Input: part model. Units: mm. Frame: model coordinates. Face numbers are marked on the shaded views. A direction names the side the tool comes from. Round coordinates to 2 decimals unless told otherwise and drop trailing zeros. Loops run counter-clockwise (first coordinate to the right, second up) from the corner with the lowest first, then second, coordinate; pieces in that order, holes last.
(1) Cut plane B-B, the plane x = 26.5. Output: boundary loops of the cut face in (y, z), and give its area (3 significant figures).
(2) Cut plane D-D, the plane x = 8. Output: boundary loops of the cut face in (y, z), and give its area (3 significant figures).
(3) Cut plane A-A, the plane z = -8.5. Output: boundary loops of the cut face in (x, y).
(4) Cut plane C-C, the plane y = 15.5. Output: boundary loops of the cut face in (x, z), and give its area (3 significant figures).
(5) First-contact query: pin 1 Ø3 at (x, y) = (25.5, 24) entering from -Z; pin 2 Ø1.5 at (y, z) = (-6.5, -18.5) entering from -X; pin 3 Ø7 at (y, z) = (22.5, -12) entering from -X. Flat tips, straight axial feed; report the tip coordinate or a pass-through.
(6) Draft query along X for the marked faces 1, 2 and 3. Return one class per face: released by +X, released by -X, zero draft, split by the parting line, or undercut.
(7) Access query for the marked faces 4, 5, 6 and 7. Directions: +Z, -Z, +X, -X, +Y, -Y. A direction counts if a zero-diameter tool reaches every point of the face in a straight line with its end or side. Return the directions, or none.
(8) Line query: line 1 (Y direction, x = 26.5, z = -3.4); line 2 (X direction, y = 7, z = -4); line 3 (X direction, y = 21.5, z = -9.75). Output: solid intervals per line, ascending.
from build123d import *

# Parameters (mm, degrees)
EXTRUDE_1_DEPTH     = 30
FILLET_1_R          = 2
SKETCH_2_W          = 4
SKETCH_2_H          = 30
EXTRUDE_2_DEPTH     = 12
SKETCH_3_W          = 79.384571865
SKETCH_3_H          = 60.739492306
CUT_EXTRUDE_1_DEPTH = 30
SKETCH_4_R          = 1.75
CUT_EXTRUDE_2_DEPTH = 30
SKETCH_5_R          = 3
CUT_EXTRUDE_3_DEPTH = 2
FILLET_2_R          = 2
SKETCH_6_W          = 24
SKETCH_6_H          = 3
EXTRUDE_4_DEPTH     = 12
SKETCH_7_R          = 1.7
CUT_EXTRUDE_4_DEPTH = 12
FILLET_3_R          = 3
FILLET_4_R          = 2


with BuildPart() as part:
    # 草图1 → 凸台-拉伸1 (new body)
    with BuildSketch(Plane(origin=(0, 0, 0), x_dir=(1, 0, 0), z_dir=(0, 1, 0))):
        with BuildLine():
            Line((15.165750888, 20.5), (-15.165750888, 20.5))
            ThreePointArc((-15.165750888, 20.5), (-18.03122292, 18.03122292), (-20.5, 15.165750888))
            Line((-20.5, 15.165750888), (-20.5, -15.165750888))
            ThreePointArc((-20.5, -15.165750888), (-18.03122292, -18.03122292), (-15.165750888, -20.5))
            Line((-15.165750888, -20.5), (15.165750888, -20.5))
            ThreePointArc((15.165750888, -20.5), (18.03122292, -18.03122292), (20.5, -15.165750888))
            Line((20.5, -15.165750888), (20.5, 15.165750888))
            ThreePointArc((20.5, 15.165750888), (18.03122292, 18.03122292), (15.165750888, 20.5))
        make_face()
        with BuildLine():
            Line((-17.5, 14.142135624), (-17.5, -14.142135624))
            ThreePointArc((-17.5, -14.142135624), (-15.909902577, -15.909902577), (-14.142135624, -17.5))
            Line((-14.142135624, -17.5), (14.142135624, -17.5))
            ThreePointArc((14.142135624, -17.5), (15.909902577, -15.909902577), (17.5, -14.142135624))
            Line((17.5, -14.142135624), (17.5, 14.142135624))
            ThreePointArc((17.5, 14.142135624), (15.909902577, 15.909902577), (14.142135624, 17.5))
            Line((14.142135624, 17.5), (-14.142135624, 17.5))
            ThreePointArc((-14.142135624, 17.5), (-15.909902577, 15.909902577), (-17.5, 14.142135624))
        make_face(mode=Mode.SUBTRACT)
    extrude(amount=EXTRUDE_1_DEPTH)

    # 圆角1
    fillet_1_edges = [part.edges().sort_by_distance(p)[0] for p in [
        (-14.142135624, 15, -17.5),
        (-17.5, 15, -14.142135624),
        (-17.5, 15, 14.142135624),
        (-14.142135624, 15, 17.5),
        (14.142135624, 15, 17.5),
        (17.5, 15, 14.142135624),
        (17.5, 15, -14.142135624),
        (14.142135624, 15, -17.5),
    ]]
    fillet(fillet_1_edges, radius=FILLET_1_R)

    # 草图2 → 凸台-拉伸2 (add)
    with BuildSketch(Plane.ZY.offset(20.5)):
        with Locations((-2.25, 15)):
            Rectangle(SKETCH_2_W, SKETCH_2_H)
    extrude_2 = extrude(amount=EXTRUDE_2_DEPTH)

    # 草图3 → 切除-拉伸1 (cut)
    with BuildSketch(Plane.XY.offset(-0.25)):
        with Locations((-5.656839026, 19.40389916)):
            Rectangle(SKETCH_3_W, SKETCH_3_H)
    cut_extrude_1 = extrude(amount=CUT_EXTRUDE_1_DEPTH, mode=Mode.SUBTRACT)

    # 草图4 → 切除-拉伸2 (cut)
    with BuildSketch(Plane(origin=(0, 0, -4.25), x_dir=(-1, 0, 0), z_dir=(0, 0, -1))):
        with Locations(Location((26.5, 23, 0), (0, 0, 90))):
            Circle(SKETCH_4_R)
        with Locations(Location((26.5, 7, 0), (0, 0, 90))):
            Circle(SKETCH_4_R)
    cut_extrude_2 = extrude(amount=-CUT_EXTRUDE_2_DEPTH, mode=Mode.SUBTRACT)

    # 草图5 → 切除-拉伸3 (cut)
    with BuildSketch(Plane(origin=(0, 0, -4.25), x_dir=(-1, 0, 0), z_dir=(0, 0, -1))):
        with Locations(Location((26.5, 23, 0), (0, 0, 90))):
            Circle(SKETCH_5_R)
        with Locations(Location((26.5, 7, 0), (0, 0, 90))):
            Circle(SKETCH_5_R)
    cut_extrude_3 = extrude(amount=-CUT_EXTRUDE_3_DEPTH, mode=Mode.SUBTRACT)

    # 镜向1: 凸台-拉伸2, 切除-拉伸1, 切除-拉伸2, 切除-拉伸3 across plane
    add(extrude_2.mirror(Plane.ZY))
    add(cut_extrude_1.mirror(Plane.ZY), mode=Mode.SUBTRACT)
    add(cut_extrude_2.mirror(Plane.ZY), mode=Mode.SUBTRACT)
    add(cut_extrude_3.mirror(Plane.ZY), mode=Mode.SUBTRACT)

    # 圆角2
    fillet_2_edges = [part.edges().sort_by_distance(p)[0] for p in [
        (-20.5, 15, -4.25),
        (-32.5, 30, -2.25),
        (-32.5, 0, -2.25),
        (17.5, 15, -0.25),
        (-17.5, 15, -0.25),
        (32.5, 0, -2.25),
        (32.5, 30, -2.25),
        (20.5, 15, -4.25),
    ]]
    fillet(fillet_2_edges, radius=FILLET_2_R)

    # 草图6 → 凸台-拉伸4 (add)
    with BuildSketch(Plane(origin=(0, 0, 0), x_dir=(1, 0, 0), z_dir=(0, 1, 0))):
        with Locations((0, 19)):
            Rectangle(SKETCH_6_W, SKETCH_6_H)
    extrude(amount=-EXTRUDE_4_DEPTH)

    # 草图7 → 切除-拉伸4 (cut)
    with BuildSketch(Plane(origin=(0, 0, -20.5), x_dir=(-1, 0, 0), z_dir=(0, 0, -1))):
        with Locations((8, -8.5)):
            Circle(SKETCH_7_R)
        with Locations(Location((-8, -8.5, 0), (0, 0, 180))):
            Circle(SKETCH_7_R)
    extrude(amount=-CUT_EXTRUDE_4_DEPTH, mode=Mode.SUBTRACT)

    # 圆角3
    fillet_3_edges = [part.edges().sort_by_distance(p)[0] for p in [
        (-12, 0, -19),
        (12, 0, -19),
    ]]
    fillet(fillet_3_edges, radius=FILLET_3_R)

    # 圆角4
    fillet_4_edges = [part.edges().sort_by_distance(p)[0] for p in [
        (-12, -12, -19),
        (12, -12, -19),
    ]]
    fillet(fillet_4_edges, radius=FILLET_4_R)


solid = part.part
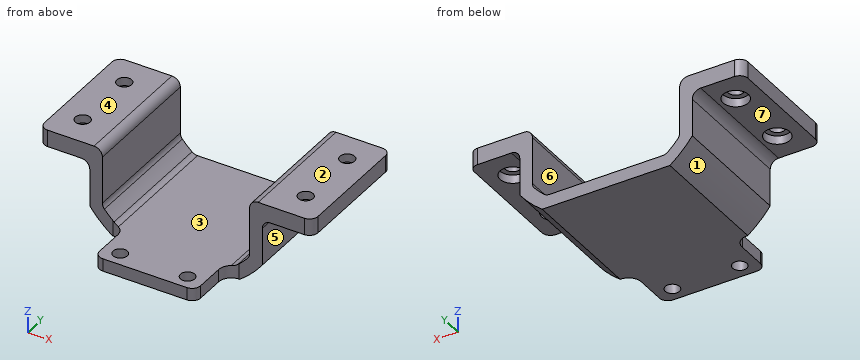
Reported:
1. outline: (0, -4.25) - (4, -4.25) - (4, -2.25) - (5.25, -2.25) - (5.25, -0.25) - (0, -0.25) - close; (8.75, -2.25) - (10, -2.25) - (10, -4.25) - (20, -4.25) - (20, -2.25) - (21.25, -2.25) - (21.25, -0.25) - (8.75, -0.25) - close; (24.75, -2.25) - (26, -2.25) - (26, -4.25) - (30, -4.25) - (30, -0.25) - (24.75, -0.25) - close
1. area: 82.0 mm2
2. outline: (-12, -20.5) - (-10.2, -20.5) - (-10.2, -17.5) - (-12, -17.5) - close; (-6.8, -20.5) - (30, -20.5) - (30, -17.5) - (-6.8, -17.5) - close
2. area: 116 mm2
3. outline: (-20.5, 0) - (-17.5, 0) - (-17.5, 30) - (-20.5, 30) - close; (17.5, 0) - (20.5, 0) - (20.5, 30) - (17.5, 30) - close
4. outline: (-32.5, -4.25) - (-22.5, -4.25) arc R2 cw to (-20.5, -6.25) - (-20.5, -15.17) arc R25.5 ccw to (-15.17, -20.5) - (15.17, -20.5) arc R25.5 ccw to (20.5, -15.17) - (20.5, -6.25) arc R2 cw to (22.5, -4.25) - (32.5, -4.25) - (32.5, -0.25) - (19.5, -0.25) arc R2 ccw to (17.5, -2.25) - (17.5, -13.42) arc R2 cw to (17.01, -14.73) arc R22.5 cw to (14.73, -17.01) arc R2 cw to (13.42, -17.5) - (-13.42, -17.5) arc R2 cw to (-14.73, -17.01) arc R22.5 cw to (-17.01, -14.73) arc R2 cw to (-17.5, -13.42) - (-17.5, -2.25) arc R2 ccw to (-19.5, -0.25) - (-32.5, -0.25) - close
4. area: 308 mm2
5. pin 1: stops at z = -2.25
5. pin 2: stops at x = -12
5. pin 3: stops at x = -20.5
6. face 1: released by -X
6. face 2: zero draft
6. face 3: undercut
7. face 4: +Z, +X, -X, +Y, -Y
7. face 5: -Z, +X, +Y, -Y
7. face 6: +Z, +Y, -Y
7. face 7: -Z, -X, +Y, -Y
8. line 1: y = 0 to 4, 10 to 20, 26 to 30
8. line 2: x = -32.5 to -29.5, -23.5 to -17.5, 17.5 to 23.5, 29.5 to 32.5
8. line 3: x = -20.5 to -17.5, 17.5 to 20.5
